from build123d import *

# Parameters (mm, degrees)
PAD001_DEPTH = 4
SKETCH_W     = 44
SKETCH_H     = 44
PAD_DEPTH    = 4
FILLET_R     = 3


with BuildPart() as body001:
    # Sketch001 → Pad001 (new body)
    with BuildSketch(Plane.XZ):
        Polygon((40, -10), (40, 25), (15, 25), (15, 4), (-15, 4), (-15, 25), (-40, 25), (-40, -10), (-23, -10), (-23, 0), (23, 0), (23, -10), align=None)
        with BuildLine():
            ThreePointArc((-33, 20), (-35, 22), (-37, 20))
            Line((-37, 20), (-37, 16))
            ThreePointArc((-37, 16), (-35, 14), (-33, 16))
            Line((-33, 20), (-33, 16))
        make_face(mode=Mode.SUBTRACT)
        with BuildLine():
            ThreePointArc((-33, -1), (-35, 1), (-37, -1))
            Line((-37, -1), (-37, -5))
            ThreePointArc((-37, -5), (-35, -7), (-33, -5))
            Line((-33, -1), (-33, -5))
        make_face(mode=Mode.SUBTRACT)
        with BuildLine():
            ThreePointArc((37, 20), (35, 22), (33, 20))
            Line((33, 20), (33, 16))
            ThreePointArc((33, 16), (35, 14), (37, 16))
            Line((37, 20), (37, 16))
        make_face(mode=Mode.SUBTRACT)
        with BuildLine():
            ThreePointArc((37, -1), (35, 1), (33, -1))
            Line((33, -1), (33, -5))
            ThreePointArc((33, -5), (35, -7), (37, -5))
            Line((37, -1), (37, -5))
        make_face(mode=Mode.SUBTRACT)
    extrude(amount=PAD001_DEPTH)


with BuildPart() as body001_1:
    # Body001 placement: moved
    add(body001.part.moved(Location((0, -22, 0))))


with BuildPart() as fillet_body:
    # Sketch → Pad (new body)
    with BuildSketch(Plane.XY):
        Rectangle(SKETCH_W, SKETCH_H)
        with BuildLine():
            ThreePointArc((-13.5, 18.5), (-15.5, 20.5), (-17.5, 18.5))
            Line((-17.5, 18.5), (-17.5, 12.5))
            ThreePointArc((-17.5, 12.5), (-15.5, 10.5), (-13.5, 12.5))
            Line((-13.5, 18.5), (-13.5, 12.5))
        make_face(mode=Mode.SUBTRACT)
        with BuildLine():
            ThreePointArc((-13.5, -12.5), (-15.5, -10.5), (-17.5, -12.5))
            Line((-17.5, -12.5), (-17.5, -18.5))
            ThreePointArc((-17.5, -18.5), (-15.5, -20.5), (-13.5, -18.5))
            Line((-13.5, -12.5), (-13.5, -18.5))
        make_face(mode=Mode.SUBTRACT)
        with BuildLine():
            ThreePointArc((17.5, 18.5), (15.5, 20.5), (13.5, 18.5))
            Line((13.5, 18.5), (13.5, 12.5))
            ThreePointArc((13.5, 12.5), (15.5, 10.5), (17.5, 12.5))
            Line((17.5, 18.5), (17.5, 12.5))
        make_face(mode=Mode.SUBTRACT)
        with BuildLine():
            ThreePointArc((17.5, -12.5), (15.5, -10.5), (13.5, -12.5))
            Line((13.5, -12.5), (13.5, -18.5))
            ThreePointArc((13.5, -18.5), (15.5, -20.5), (17.5, -18.5))
            Line((17.5, -12.5), (17.5, -18.5))
        make_face(mode=Mode.SUBTRACT)
        with BuildLine():
            ThreePointArc((12, 3), (0, 15), (-12, 3))
            Line((-12, 3), (-12, -3))
            ThreePointArc((-12, -3), (0, -15), (12, -3))
            Line((12, 3), (12, -3))
        make_face(mode=Mode.SUBTRACT)
    extrude(amount=PAD_DEPTH)

    # Fusion001: union Body001
    add(body001_1.part)

    # Fillet
    fillet_edges = [fillet_body.edges().sort_by_distance(p)[0] for p in [
        (-22, 22, 2),
        (22, 22, 2),
        (-23, -24, -10),
        (-40, -24, -10),
        (-40, -24, 25),
        (-15, -24, 25),
        (23, -24, -10),
        (40, -24, -10),
        (15, -24, 25),
        (40, -24, 25),
    ]]
    fillet(fillet_edges, radius=FILLET_R)


solid = fillet_body.part
Could you check a few things on this model? Use its own coordinates, in mm. A direction names the side the tool comes from. Coordinates: 2 decimals unless noted, no trailing zeros. Order: outer loops, then holes, each group sorted by start corner. A loop starts at its lowest first (then second) coordinate and runs counter-clockwise, first axis right, second up. Notation, with made-up numbers: (13.25, -12.5) -> (35.25, -12.5) arc R12 cw to (35.25, -0.5) -> close; hole circle Ø10 at (42, -35). An arc over 180 degrees is marked (long way). One line per item, written item: value. Start each with the question number.
1) We'd pull the mould along X, two halves only. Please class faces 1 (the flat face through (40, -24, 7)), 2 (the flat face through (-33, -24, -3)), 3 (the flat face through (28, -24, 25)), 4 (the flat face through (12, 0, 2)): +X half, -X half, draft (parallel to the pull), parting line (faces both ways), or undercut.
2) Imagine slicing it at B-B on y = 4.5. List the corners of the cut face in (x, z) for me, plus the area to 3 significant figures.
3) Imagine slicing it at C-C on x = 29.5. List the corners of the cut face in (y, z) for me, plus the area to 3 significant figures.
4) If I drill on L1, parallel to Z at x = -20.5, y = 4.5; L2, parallel to Y at x = -23, z = 23.5; L3, parallel to X at y = 13.5, z = 3, over which ranges is the centre line in solid material (lowest first)? Write a range as [from, to].
5) I'm going to push flat-ended pins straight in: pin 1 (22 mm diameter, centred on x = -6, y = 7.5, fed in from +Z); pin 2 (1.5 mm diameter, centred on x = -25, y = -19.5, fed in from -Z); pin 3 (10 mm diameter, centred on y = -9, z = 0.5, fed in from -X); pin 4 (1.2 mm diameter, centred on y = 16.5, z = 2, fed in from +X). Where does each tip first touch, or does it pass through?
6) Which directions (+Z, -Z, +X, -X, +Y, -Y) give clear straight access to the entire face, cutting with the end or side of a thin tool? Please do faces 5 (the cylindrical face through (15.9, -24.03, 24.14)), 6 (the flat face through (-23, -24, -4)), 7 (the flat face through (37, -24, 18)), 8 (the cylindrical face through (39.14, -24.03, 24.1)), 9 (the cylindrical face through (-15.5, -10.5, 2)).
7) Imagine slicing it at A-A on z = 11.5. List the corners of the cut face in (x, y) for me.
Answer list:
1. face 1: +X half
1. face 2: undercut
1. face 3: draft
1. face 4: undercut
2. outline: (-22, 0) -> (-11.91, 0) -> (-11.91, 4) -> (-22, 4) -> close; (11.91, 0) -> (22, 0) -> (22, 4) -> (11.91, 4) -> close
2. area: 80.8 mm2
3. outline: (-26, -10) -> (-22, -10) -> (-22, 25) -> (-26, 25) -> close
3. area: 140 mm2
4. L1: z = [0, 4]
4. L2: y = [-26, -22]
4. L3: x = [-22, -17.5], [-13.5, -5.81], [5.81, 13.5], [17.5, 22]
5. pin 1: stops at z = 4
5. pin 2: passes through
5. pin 3: stops at x = -22
5. pin 4: stops at x = 22
6. face 5: +Z, +Y, -Y
6. face 6: -Z, +Y, -Y
6. face 7: +Y, -Y
6. face 8: +Z, +X, +Y, -Y
6. face 9: +Z, -Z
7. outline: (-40, -26) -> (-15, -26) -> (-15, -22) -> (-40, -22) -> close; (15, -26) -> (40, -26) -> (40, -22) -> (15, -22) -> close
